Geometry check sheet. Reference: the model listing, model coordinates, mm. Face numbers are marked on the shaded views. A direction names the side the tool comes from. Coordinates: 2 decimals unless noted, no trailing zeros. Write each loop counter-clockwise with the first axis right and the second up, starting at its lowest first coordinate (ties: lowest second). Pieces come first, ordered by that corner, then holes. Notation, with made-up numbers: (13, -14) -> (28, -14) arc R32 ccw to (28, 12) -> close; hole circle Ø2 at (24, -23). An arc over 180 degrees is marked (long way). Answer in a Markdown table with one row per item. Add a question column.
1. Scan lines: L1, parallel to Z at x = -4.5, y = 7; L2, parallel to X at y = 3.4, z = 2.4; L3, parallel to Y at x = -3.4, z = -5.25. Record each from-to range of solid material in increasing order. Write a range as from..to.
2. Cross-section at C-C on x = 8. Record the cut outline in (y, z), and give its area (3 significant figures).
3. Cross-section at D-D on z = -32. Record the cut outline in (x, y).
4. Depth check by flat-ended pin: P1, Ø5, axis at y = 17, z = 27.5, coming from the -X side; P2, Ø6, axis at x = -1.5, y = 28, coming from the +Z side; P3, Ø2, axis at x = 2, y = 31, coming from the +Z side. Enter the tip coordinate at first touch or a pass-through.
5. Set-up check for the marked faces 5, 6 and 7: record each of +Z, -Z, +X, -X, +Y, -Y from which the full face is reachable in a straight line by a thin tool's end or side.
6. Cross-section at A-A on z = 2. Record the cut outline in (x, y), and give its area (3 significant figures).
7. Mould release check, pull along Z, two halves, no side actions. Record for the marked faces 1, 2, 3 and 4: pulls with the +Z half, pulls with the -Z half, needs draft (parallel to the pull), parting line crosses it, or undercut.
8. Cross-section at B-B on y = 27. Record the cut outline in (x, z).
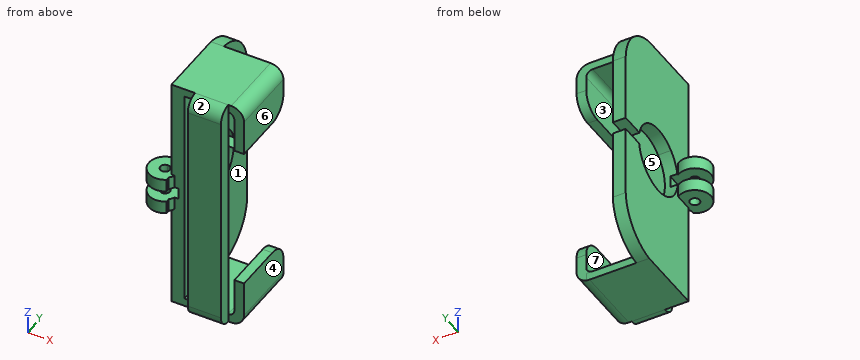
Autodesk Inventor part; units mm, degrees
ref_plane "YZ Plane" through (0, 0, 0) normal (1, 0, 0) x (0, 1, 0)
ref_plane "XZ Plane" through (0, 0, 0) normal (0, 1, 0) x (-1, 0, 0)
ref_plane "XY Plane" through (0, 0, 0) normal (0, 0, 1) x (1, 0, 0)
sketch "Эскиз1" plane through (0, 0, 0) normal (0, 0, 1) x (1, 0, 0)
  arc A0 (-3.5681, 4.8905) -> (-4.8473, 3.794) centre (-3.4, 3.4) ccw
  circle A1 centre (-3.4, 3.4) radius 1.5
  arc A2 (0.4144, 4.9) -> (0.4144, 1.9) centre (-3.4, 3.4) ccw
  line L0 (0.4144, 4.9) -> (0.4144, 1.9)
  point P0 (0, 0)
  point P1 (-4.8473, 3.794)
  point P2 (-3.5681, 4.8905)
extrude "Выдавливание1" add sketch "Эскиз1" along normal blind 4
sketch "Эскиз2" plane through (0.4144, 1.9, 0) normal (1, 0, 0) x (0, 0, -1)
  line L0 (0, 0) -> (0, 3)
  line L1 (0, 3) -> (-4, 3)
  line L2 (-4, 0) -> (-4, 3)
  line L3 (0, 0) -> (-4, 0)
  line L4 (0, 3) -> (-4, 3)
  line L5 (-4, 3) -> (7.5, 3)
  line L6 (7.5, 3) -> (7.5, 0)
  line L7 (7.5, 0) -> (-4, 0)
  line L8 (-4, 0) -> (-4, 3)
  point P0 (0, -1.9)
  point P1 (3, 1.9)
  dimension "d2" = 4
  dimension "d3" = 4.5
extrude "Выдавливание2" add sketch "Эскиз2" along normal blind 3
sketch "Эскиз3" plane through (0.4144, 1.9, -7.5) normal (0, 0, -1) x (-1, 0, 0)
  line L0 (0, 0) -> (0, 3)
  arc A0 (0, 0) -> (0, 3) centre (3.8144, 1.5) ccw
  circle A1 centre (3.8144, 1.5) radius 1.5
  point P0 (0.4144, -1.9)
extrude "Выдавливание3" add sketch "Эскиз3" against normal blind 4
sketch "Эскиз4" plane through (3.4144, 1.9, 0) normal (1, 0, 0) x (0, 0, -1)
  line L0 (6.3383, 0) -> (-1.6617, 0)
  line L1 (39.5883, 0) -> (-34.9117, 0)
  line L2 (-34.9117, 0) -> (-34.9117, 21.3)
  line L3 (-21.0745, 33.9845) -> (25.7512, 33.9845)
  line L4 (39.5883, 21.3002) -> (39.5883, 0)
  line L5 (-31.9117, 21.3) -> (-31.9117, 4.3)
  line L6 (36.5883, 4.3) -> (36.5883, 21.3)
  line L7 (24.5883, 33.3) -> (-19.9117, 33.3)
  arc A0 (-19.9117, 33.9845) -> (-34.9117, 21.3) centre (-20.4931, 19.4607) ccw
  circle A1 centre (2.3383, 16.3) radius 0.9967
  line L8 (2.3383, 16.3) -> (2.3383, 42.847) construction
  arc A2 (39.5883, 21.3) -> (24.5883, 33.9845) centre (25.1697, 19.4607) ccw
  point P0 (0, -1.9)
  point P1 (-1.6617, 0)
  dimension "d8" = 3
  dimension "d9" = 3
extrude "Выдавливание4" add sketch "Эскиз4" against normal blind 4 contours L0 L1 L2 A0 L3 A2 L4
sketch "Эскиз5" plane through (-0.5856, 1.9, 0) normal (-1, 0, 0) x (0, 0, 1)
  arc A0 (-10.3389, 9.5) -> (5.6623, 9.5) centre (-2.3383, 16.3) ccw
  circle A1 centre (-2.3383, 16.3) radius 0.9967
  circle A2 centre (-2.3383, 16.3) radius 10.5
  point P0 (0, -1.9)
  point P1 (5.6623, 9.5)
  point P2 (-10.3389, 9.5)
extrude "Выдавливание5" cut sketch "Эскиз5" against normal blind 4
sketch "Эскиз6" plane through (3.4144, 1.9, 0) normal (1, 0, 0) x (0, 0, -1)
  circle A0 centre (2.3383, 16.3) radius 10.5
  line L0 (-34.9117, 0) -> (39.5883, 0)
  line L1 (39.5883, 0) -> (39.5883, 21.3002)
  arc A1 (39.5883, 21.3002) -> (25.7512, 33.9845) centre (25.1697, 19.4607) ccw
  line L2 (25.7512, 33.9845) -> (-21.0745, 33.9845)
  arc A2 (-21.0745, 33.9845) -> (-34.9117, 21.3) centre (-20.4931, 19.4607) ccw
  line L3 (-34.9117, 21.3) -> (-34.9117, 0)
  line L4 (-34.9117, 0) -> (-32.4117, 0)
  line L5 (-32.4117, 0) -> (-32.4117, 21.3)
  line L6 (-32.4117, 21.3) -> (-34.9117, 21.3)
  line L7 (-34.9117, 21.3) -> (-34.9117, 0)
  line L8 (39.5883, 0) -> (39.5883, 21.3002)
  line L9 (39.5883, 0) -> (37.0883, 0)
  line L10 (37.0883, 0) -> (37.0883, 21.3)
  line L11 (37.0883, 21.3) -> (39.5883, 21.3)
  line L12 (39.5883, 21.3) -> (39.5883, 0)
  point P0 (0, -1.9)
  dimension "d14" = 2.5
  dimension "d15" = 2.5
extrude "Выдавливание6" add sketch "Эскиз6" along normal blind 15.5 contours L3 L6 L5 L0 | L10 L11 L1 L0
sketch "Эскиз7" plane through (-0.5856, 1.9, 0) normal (-1, 0, 0) x (0, 0, 1)
  circle A0 centre (-2.3383, 16.3) radius 10.5
  line L0 (-3.82, 35.4662) -> (0, 35.4662)
  line L1 (0, 35.4662) -> (0, 24.6625)
  line L2 (0, 24.6625) -> (-3.82, 24.6625)
  line L3 (-3.82, 24.6625) -> (-3.82, 35.4662)
  point P0 (0, -1.9)
  point P1 (-3.82, 26.6949)
  point P2 (0, 26.5363)
extrude "Выдавливание7" cut sketch "Эскиз7" against normal blind 15.5 contours A0 L3 L0 L1
sketch "Эскиз8" plane through (0.4144, 1.9, 0) normal (0, -1, 0) x (1, 0, 0)
  line L0 (3, 32.4117) -> (18.5, 32.4117)
  line L1 (3, -37.0883) -> (18.5, -37.0883)
  line L2 (16.6252, 32.4117) -> (6.3462, 32.4117)
  line L3 (6.3462, 32.4117) -> (6.3462, -37.0883)
  line L4 (6.3462, -37.0883) -> (16.6252, -37.0883)
  line L5 (16.6252, -37.0883) -> (16.6252, 32.4117)
  line L6 (18.5, 34.9117) -> (-1, 34.9117)
  line L7 (16.6252, 34.9117) -> (6.3462, 34.9117)
  line L8 (6.3462, 34.9117) -> (6.3462, 32.4117)
  line L9 (6.3462, 32.4117) -> (16.6252, 32.4117)
  line L10 (16.6252, 32.4117) -> (16.6252, 34.9117)
  line L11 (-1, -39.5883) -> (18.5, -39.5883)
  line L12 (16.6252, -37.0883) -> (6.3462, -37.0883)
  line L13 (6.3462, -37.0883) -> (6.3462, -39.5883)
  line L14 (6.3462, -39.5883) -> (16.6252, -39.5883)
  line L15 (16.6252, -39.5883) -> (16.6252, -37.0883)
  point P0 (-0.4144, 0)
  point P1 (6.3462, -37.0883)
extrude "Выдавливание8" add sketch "Эскиз8" along normal blind 4
fillet "Сопряжение1" radius 4 2 edges at (11.9001, -2.1, -39.5883) (11.9001, -2.1, 34.9117)
sketch "Эскиз9" plane through (18.9144, 1.9, -39.5883) normal (0, -1, 0) x (1, 0, 0)
  line L0 (-15.5, 74.5) -> (0, 74.5)
  line L1 (0, 74.5) -> (3, 74.5)
  line L2 (3, 74.5) -> (3, 59.5)
  line L3 (3, 59.5) -> (0, 59.5)
  line L4 (0, 59.5) -> (0, 74.5)
  line L5 (0, 2.5) -> (0, 0)
  line L6 (0, 0) -> (3, 0)
  line L7 (3, 0) -> (3, 15)
  line L8 (3, 15) -> (0, 15)
  line L9 (0, 15) -> (0, 0)
  point P0 (-18.9144, 39.5883)
  dimension "d23" = 3
  dimension "d24" = 15
  dimension "d25" = 15
extrude "Выдавливание9" add sketch "Эскиз9" against normal blind 21.3
fillet "Сопряжение2" radius 4 2 edges at (21.9144, 12.55, -39.5883) (21.9144, 12.55, 34.9117)
fillet "Сопряжение3" radius 2 2 edges at (18.9144, 12.55, 32.4117) (18.9144, 12.55, -37.0883)
fillet "Сопряжение4" radius 6 2 edges at (20.4144, 23.2, 19.9117) (20.4144, 23.2, -24.5883)
sketch "Эскиз10" plane through (0.4144, 1.9, -7.5) normal (0, 0, -1) x (-1, 0, 0)
  circle A0 centre (3.8144, 1.5) radius 1.5
  arc A1 (0, 0) -> (1, 4.4797) centre (3.8144, 1.5) ccw
  arc A2 (1, -2.6327) -> (1, 5.6327) centre (3.8144, 1.5) ccw
  line L0 (1, 0) -> (1, 21.3)
  line L1 (1, 6.5) -> (1, -2.6327)
  point P0 (0.4144, -1.9)
  point P1 (1, -1.4797)
  dimension "d31" = 10
extrude "Выдавливание10" add sketch "Эскиз10" against normal blind 4 contours A1 L0 A2 L1
sketch "Эскиз11" plane through (0, 0, 4) normal (0, 0, 1) x (1, 0, 0)
  arc A0 (-0.5856, 7.5327) -> (-0.5856, -0.7327) centre (-3.4, 3.4) ccw
  circle A1 centre (-3.4, 3.4) radius 1.5
  circle A2 centre (-3.4, 3.4) radius 5
  line L0 (-0.5856, 1.9) -> (-0.5856, 7.5327)
  line L1 (-0.5856, 7.5327) -> (-0.5856, -0.7327)
  circle A3 centre (-3.4, 3.4) radius 1.5
  line L2 (0.4144, 1.9) -> (-0.5856, 1.9)
  line L3 (-0.5856, 1.9) -> (-0.5856, 6.3797)
  arc A4 (-0.5856, 6.3797) -> (0.4144, 1.9) centre (-3.4, 3.4) ccw
  point P0 (0, 0)
  point P1 (-0.5856, 0.4203)
extrude "Выдавливание11" add sketch "Эскиз11" against normal blind 4 contours L0 A4 L1 A0
sketch "Эскиз12" plane through (0.4144, -2.1, 0) normal (0, -1, 0) x (1, 0, 0)
  line L0 (-1, -3.5) -> (-1, 0)
  line L1 (3, 0) -> (-1, 0)
  line L2 (-1, 0) -> (1.1974, 0)
  line L3 (1.1974, 0) -> (1.1974, -3.5)
  line L4 (1.1974, -3.5) -> (-1, -3.5)
  line L5 (-1, -3.5) -> (-1, 0)
  point P0 (-0.4144, 0)
extrude "Выдавливание12" cut sketch "Эскиз12" against normal blind 21.5
properties part number "cam_hold_logitech"
Results found:
| question | item | result |
|---|---|---|
| 1 | L1 | z = -7.5..-3.5, 0..4 |
| 1 | L2 | x = -8.4..-4.9, -1.9..3.41 |
| 1 | L3 | y = -1.6..1.9, 4.9..8.4 |
| 2 | outline | (-2.1, -35.59) arc R4 ccw to (1.9, -39.59) -> (23.2, -39.59) -> (23.2, -37.09) -> (1.9, -37.09) -> (1.9, 32.41) -> (23.2, 32.41) -> (23.2, 34.91) -> (1.9, 34.91) arc R4 ccw to (-2.1, 30.91) -> close |
| 2 | area | 398 mm^2 |
| 3 | outline | (-0.59, 1.9) -> (3.41, 1.9) -> (3.41, 34.19) -> (-0.59, 34.19) -> close; (6.76, -2.1) -> (17.04, -2.1) -> (17.04, 1.9) -> (6.76, 1.9) -> close; (18.91, 1.9) -> (21.91, 1.9) -> (21.91, 23.2) -> (18.91, 23.2) -> close |
| 4 | P1 | stops at x = -0.59 |
| 4 | P2 | stops at z = 34.53 |
| 4 | P3 | stops at z = 32.18 |
| 5 | face 5 | +Y |
| 5 | face 6 | +Z, -Z, +X, +Y, -Y |
| 5 | face 7 | +Y, -Y |
| 6 | outline | (-0.59, -0.73) -> (-0.59, 0.42) arc R4.1 ccw to (0.41, 1.9) -> (3.41, 1.9) -> (3.41, 8.64) -> (-0.59, 8.64) -> (-0.59, 7.53) arc R5 ccw (long way) to start; (-0.59, 27.76) -> (3.41, 27.76) -> (3.41, 35.88) -> (-0.59, 35.88) -> close; (6.76, -2.1) -> (17.04, -2.1) -> (17.04, 1.9) -> (6.76, 1.9) -> close; hole (-4.85, 3.79) arc R1.5 ccw (long way) to (-3.57, 4.89) arc R1.5 ccw to start |
| 6 | area | 160 mm^2 |
| 7 | face 1 | undercut |
| 7 | face 2 | pulls with the +Z half |
| 7 | face 3 | undercut |
| 7 | face 4 | needs draft |
| 8 | outline | (-0.59, -38.57) -> (3.41, -38.57) -> (3.41, -8.07) -> (-0.59, -8.07) -> close; (-0.59, 3.39) -> (3.41, 3.39) -> (3.41, 33.89) -> (-0.59, 33.89) -> close |
